Could you check a few things on this model? Use its own coordinates, in mm. A direction names the side the tool comes from. Coordinates: 2 decimals unless noted, no trailing zeros. Loops run counter-clockwise (first coordinate to the right, second up) from the corner with the lowest first, then second, coordinate; pieces in that order, holes last.
1) Thinking about a two-plate mould opening in X: for faces 1 (the face through (363, 198, -25)), 2 (the face through (943.986, 5.703, 0.35)), 3 (the face through (471, 100, 0)), which applies, released by +X, released by -X, zero draft, split by the parting line, or undercut?
2) If I drill on line 1 along Y through (x, z) = (100, -8); line 2 along Y through (x, z) = (350, -4); line 3 along Y through (x, z) = (341.5, -10.5), over which ranges is the centre line in solid material (lowest first)?
3) Imagine slicing it at C-C on y = 250. Please give me the cut outline in (x, z), plus the area to 3 significant figures.
4) Imagine slicing it at B-B on z = 13. Please give me the cut outline in (x, y).
5) For faces 4 (the face through (305, 400, 0)), 5 (the face through (6.014, 494.297, 0.35)), 6 (the face through (743.986, 94.297, 0.35)), which set-ups out of +Z, -Z, +X, -X, +Y, -Y let a thin tool reach every point of the face, with its end or its side?
6) Will these pins go through, and if not, where does the flat tip stop? P1, Ø4, axis at x = 188, z = -10.5, coming from the -Y side; P2, Ø6, axis at y = 254.5, z = -19.5, coming from the +X side; P3, Ø4, axis at x = 741, z = 14.5, coming from the -Y side.
7) Imagine slicing it at D-D on x = 500.5. Please give me the cut outline in (y, z), plus the area to 3 significant figures.
8) Imagine slicing it at A-A on x = 350. Please give me the cut outline in (y, z), plus the area to 3 significant figures.
```python
from build123d import *

# Parameters (mm, degrees)
BOSS_EXTRUDE4_DEPTH = 25
SKETCH8_R           = 30
SKETCH8_R_2         = 40
SKETCH8_R_3         = 25
CUT_EXTRUDE2_DEPTH  = 51


with BuildPart() as part:
    # Sketch6 → Boss-Extrude4 (new body, symmetric)
    with BuildSketch(Plane.XY):
        with BuildLine():
            Line((20, 0), (180, 0))
            ThreePointArc((180, 0), (194.142135624, 5.857864376), (200, 20))
            Line((200, 20), (200, 80))
            ThreePointArc((200, 80), (205.857864376, 94.142135624), (220, 100))
            Line((220, 100), (730, 100))
            ThreePointArc((730, 100), (744.142135624, 94.142135624), (750, 80))
            Line((750, 80), (750, 20))
            ThreePointArc((750, 20), (755.857864376, 5.857864376), (770, 0))
            Line((770, 0), (930, 0))
            ThreePointArc((930, 0), (944.142135624, 5.857864376), (950, 20))
            Line((950, 20), (950, 180))
            ThreePointArc((950, 180), (944.142135624, 194.142135624), (930, 200))
            Line((930, 200), (734.664010614, 200))
            ThreePointArc((734.664010614, 200), (544.664010614, 250.910346562), (405.574357176, 390))
            ThreePointArc((405.574357176, 390), (398.2538491, 397.320508076), (388.2538491, 400))
            Line((388.2538491, 400), (220, 400))
            ThreePointArc((220, 400), (205.857864376, 405.857864376), (200, 420))
            Line((200, 420), (200, 480))
            ThreePointArc((200, 480), (194.142135624, 494.142135624), (180, 500))
            Line((180, 500), (20, 500))
            ThreePointArc((20, 500), (5.857864376, 494.142135624), (0, 480))
            Line((0, 480), (0, 20))
            ThreePointArc((0, 20), (5.857864376, 5.857864376), (20, 0))
        make_face()
    extrude(amount=BOSS_EXTRUDE4_DEPTH, both=True)

    # Sketch8 → Cut-Extrude2 (cut, through all)
    with BuildSketch(Plane.XY.offset(25)):
        with Locations((100, 400)):
            Circle(SKETCH8_R)
        with Locations((100, 100)):
            Circle(SKETCH8_R_2)
        with Locations((350, 250)):
            Circle(SKETCH8_R_3)
        with Locations((832.332005307, 100)):
            Circle(SKETCH8_R_2)
    extrude(amount=-CUT_EXTRUDE2_DEPTH, mode=Mode.SUBTRACT)


solid = part.part
```
Filled in:
1. face 1: zero draft
1. face 2: released by +X
1. face 3: undercut
2. line 1: y = 0 to 60, 140 to 370, 430 to 500
2. line 2: y = 100 to 225, 275 to 400
2. line 3: y = 100 to 226.49, 273.51 to 400
3. outline: (0, -25) - (325, -25) - (325, 25) - (0, 25) - close; (375, -25) - (546.25, -25) - (546.25, 25) - (375, 25) - close
3. area: 24,800 mm2
4. outline: (0, 20) arc R20 ccw to (20, 0) - (180, 0) arc R20 ccw to (200, 20) - (200, 80) arc R20 cw to (220, 100) - (730, 100) arc R20 cw to (750, 80) - (750, 20) arc R20 ccw to (770, 0) - (930, 0) arc R20 ccw to (950, 20) - (950, 180) arc R20 ccw to (930, 200) - (734.66, 200) arc R380 cw to (405.57, 390) arc R20 ccw to (388.25, 400) - (220, 400) arc R20 cw to (200, 420) - (200, 480) arc R20 ccw to (180, 500) - (20, 500) arc R20 ccw to (0, 480) - close; hole circle Ø80 at (100, 100); hole circle Ø60 at (100, 400); hole circle Ø50 at (350, 250); hole circle Ø80 at (832.33, 100)
5. face 4: +Z, -Z, +X, +Y
5. face 5: +Z, -Z, -X, +Y
5. face 6: +Z, -Z, -Y
6. P1: stops at y = 0.92
6. P2: stops at x = 543.65
6. P3: stops at y = 95.2
7. outline: (100, -25) - (280.72, -25) - (280.72, 25) - (100, 25) - close
7. area: 9,040 mm2
8. outline: (100, -25) - (225, -25) - (225, 25) - (100, 25) - close; (275, -25) - (400, -25) - (400, 25) - (275, 25) - close
8. area: 12,500 mm2
